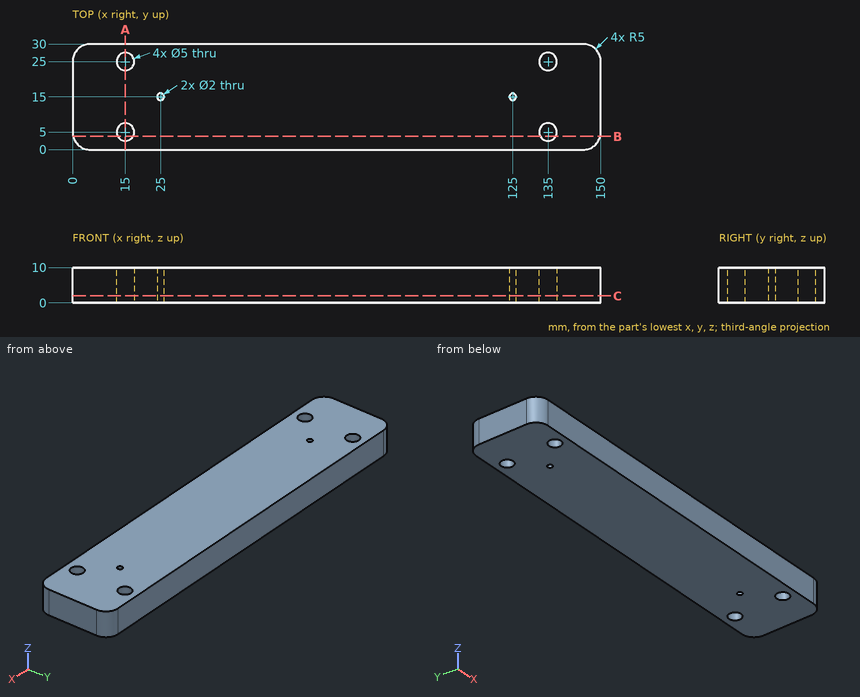
Design review of the part shown in the three views and the two pictorial views. Dimensions are in mm from the part's minimum x, y and z. Round coordinates to 2 decimals unless told otherwise and drop trailing zeros. Order: outer loops, then holes, each group sorted by start corner. A loop starts at its lowest first (then second) coordinate and runs counter-clockwise, first axis right, second up.
Item 1: Add section A-A, the plane x = 15. State the section outline as (y, z) points.
Working result:
outline: (0, 0) - (2.5, 0) - (2.5, 10) - (0, 10) - close; (7.5, 0) - (22.5, 0) - (22.5, 10) - (7.5, 10) - close; (27.5, 0) - (30, 0) - (30, 10) - (27.5, 10) - close
Item 2: For pin 1 (4.5 mm diameter, centred on x = 15, y = 25, fed in from -Z), flat-tipped, find the tip position at first contact; note if it passes through.
Working result:
pin 1: passes through
Item 3: Add section C-C, the plane z = 2. State the section outline as (x, y) points, and give its area (3 significant figures).
Working result:
outline: (0, 5) arc R5 ccw to (5, 0) - (145, 0) arc R5 ccw to (150, 5) - (150, 25) arc R5 ccw to (145, 30) - (5, 30) arc R5 ccw to (0, 25) - close; hole circle Ø5 at (15, 5); hole circle Ø5 at (15, 25); hole circle Ø2 at (25, 15); hole circle Ø2 at (125, 15); hole circle Ø5 at (135, 5); hole circle Ø5 at (135, 25)
area: 4,390 mm2
Item 4: To check wall thickness, follow probe 1 along Y at (x, z) = (135, 6); probe 2 along Y at (x, z) = (25, 3); probe 3 along X at (y, z) = (4.5, 1). State the ranges of each line that lie inside material, in increasing order.
Working result:
probe 1: y = 0 to 2.5, 7.5 to 22.5, 27.5 to 30
probe 2: y = 0 to 14, 16 to 30
probe 3: x = 0.03 to 12.55, 17.45 to 132.55, 137.45 to 149.97
Item 5: Add section B-B, the plane y = 3.75. State the section outline as (x, z) points.
Working result:
outline: (0.16, 0) - (12.83, 0) - (12.83, 10) - (0.16, 10) - close; (17.17, 0) - (132.83, 0) - (132.83, 10) - (17.17, 10) - close; (137.17, 0) - (149.84, 0) - (149.84, 10) - (137.17, 10) - close
